Can you work these out from the drawing? Everything is in mm from the part's minimum corner. Round coordinates to 2 decimals unless told otherwise and drop trailing zeros. Order: outer loops, then holes, each group sorted by start corner. A loop starts at its lowest first (then second) coordinate and runs counter-clockwise, first axis right, second up. Notation, with made-up numbers: (-11, -2) -> (-3, -2) arc R13 cw to (-3, 17) -> close; hole circle Ø10 at (-7.5, -14.5). An arc over 180 degrees is marked (long way). One line per item, written item: value.
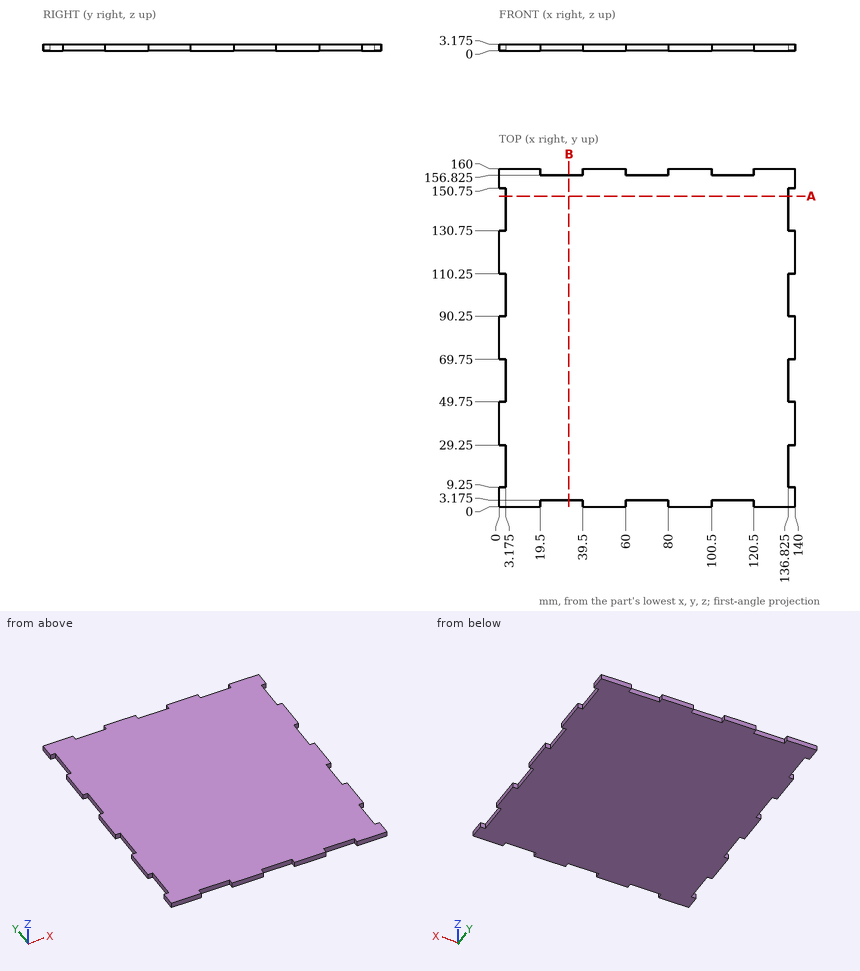
Q1. I want a section at B-B on x = 33. Write out the boundary of the cut face in (y, z) (3 decimals), then the cut area to 3 significant figures.
Answers:
outline: (3.175, 0) -> (156.825, 0) -> (156.825, 3.175) -> (3.175, 3.175) -> close
area: 488 mm2
Q2. I need wall thicknesses on line 1 along X through (y, z) = (18, 2.8) (3 decimals); line 2 along Y through (x, z) = (64.5, 2.8) (3 decimals). Which ranges of each line are inside material? Lowest first, please.
Answers:
line 1: 3.175 to 136.825
line 2: 3.175 to 156.825
Q3. I want a section at A-A on y = 147. Write out the boundary of the cut face in (x, z) (3 decimals), then the cut area to 3 significant figures.
Answers:
outline: (3.175, 0) -> (136.825, 0) -> (136.825, 3.175) -> (3.175, 3.175) -> close
area: 424 mm2
Q4. For P1, Ø1, axis at x = 111.5, z = 2, coming from the -Y side (3 decimals); P2, Ø1.6, axis at y = 14.5, z = 1, coming from the +X side (3 decimals); P3, Ø1.6, axis at x = 109.5, z = 2, coming from the +Y side (3 decimals), each with a flat end and sliding along its axis, tell me the tip position at first contact or that it passes through.
Answers:
P1: y = 3.175
P2: x = 136.825
P3: y = 156.825
